For this review, take the finished solid that the model builds, in its own axes (mm). A direction names the side the tool comes from. Give positions to 0.01 mm unless a question says otherwise; leave off trailing zeros. Write each loop counter-clockwise with the first axis right and the second up, starting at its lowest first coordinate (ties: lowest second). Pieces come first, ordered by that corner, then holes.
1) We need section B-B on z = -9. Give the boundary of the cut face in (x, y).
2) Draft analysis for pull direction Z (two halves, no side actions). For faces 3 (the face through (4, 3, 0)), 4 (the face through (0, 4, 0)), 5 (the face through (1.014, -12.956, 5.122)), 6 (the face through (4.056, 10.648, -13.887)), state which applies: pulls with the +Z half, pulls with the -Z half, needs draft (parallel to the pull), parting line crosses it, or undercut.
3) Machinability: for faces 1 (the face through (1.014, 13.492, 3.472)), 2 (the face through (5.042, -15.368, -2.018)), which of the approach directions +Z, -Z, +X, -X, +Y, -Y give a long, thin tool a straight path to every point of the face, cutting with its end or side? Answer none if there is none.
4) For P1, Ø5, axis at y = -5.88, z = -8.09, coming from the -X side; P2, Ø1.5, axis at x = 6, z = -8, coming from the -Y side; P3, Ø5, axis at y = -2.5, z = 11.5, coming from the +X side; P4, Ø1, axis at x = 3.5, z = -2, coming from the +Y side, all flat-tipped, find the tip position at first contact; note any pin that passes through.
5) We need section C-C on x = 1. Give the boundary of the cut face in (y, z).
6) We need section A-A on y = 0. Give the number of separate pieces and of enclosed holes in the cut face, and give its area (3 significant figures).
7) Wall thickness on line 1 along Y through (x, z) = (3.75, 0); line 2 along Y through (x, z) = (2.25, -4.5): over which ranges is each line inside the solid? List them lowest first.
from build123d import *

# Parameters (mm, degrees)
F0_W            = 8
F0_H            = 17.5
F3_D            = 6
F4_T            = -2
F6_D            = 8
F6_COPIES_COUNT = 5
F7_SIZE         = 0.99999


# Not quite as in the source:
# - a fillet or chamfer is up to 0.001 mm smaller than in the source, because OpenCascade refuses the exact size
# - a pattern or mirror of a feature is missing from the dataset's text; its kind, count and spacing are read off the source's solid


with BuildPart() as f1:
    # F0 (on Front) → F1 (revolve)
    with BuildSketch(Plane.XZ):
        with Locations((4, 8.75)):
            Rectangle(F0_W, F0_H)
    revolve(axis=Axis((4, 0, 0), (1, 0, 0)))

    # F3 (through all)
    with Locations(Plane(origin=(0, 0, 0), x_dir=(0, 1, 0), z_dir=(-1, 0, 0))):
        with Locations((0, 0)):
            Hole(F3_D / 2)

    # F4
    f4_openings = [f1.faces().sort_by_distance(p)[0] for p in [
        (8, 0, -17.005025),
    ]]
    offset(amount=F4_T, openings=f4_openings)

    # F6 (through all)
    with Locations(Plane(origin=(0, 0, 0), x_dir=(0, 1, 0), z_dir=(-1, 0, 0))):
        with Locations((0, -10)):
            f6 = Hole(F6_D / 2)

    # F6_copies: F6 ×5 about axis
    f6_copies_axis = Axis((0, 0, 0), (1, 0, 0))
    for i in range(1, F6_COPIES_COUNT):
        add(f6.rotate(f6_copies_axis, i * 360 / F6_COPIES_COUNT), mode=Mode.SUBTRACT)

    # F7 (size 1 in the source; OpenCascade refuses exactly that, so slightly less here)
    f7_edges = [f1.edges().sort_by_distance(p)[0] for p in [
        (8, -3, 0),
        (8, -5, 0),
    ]]
    chamfer(f7_edges, length=F7_SIZE)


solid = f1.part
Results list:
1. outline: (0, -15.01) - (8, -15.01) - (8, -12.62) - (2, -12.62) - (2, -9.77) - (0, -9.77) - close; (0, -1.98) - (2, -1.98) - (2, 1.98) - (0, 1.98) - close; (0, 9.77) - (2, 9.77) - (2, 12.62) - (8, 12.62) - (8, 15.01) - (0, 15.01) - close
2. face 3: undercut
2. face 4: needs draft
2. face 5: undercut
2. face 6: parting line crosses it
3. face 1: +X, -X
3. face 2: +X
4. P1: passes through
4. P2: stops at y = -15.93
4. P3: stops at x = 2
4. P4: stops at y = 17.44
5. outline: circle Ø35 at (0, 0); hole circle Ø8 at (-9.51, 3.09); hole circle Ø8 at (-5.88, -8.09); hole circle Ø8 at (0, 10); hole circle Ø6 at (0, 0); hole circle Ø8 at (5.88, -8.09); hole circle Ø8 at (9.51, 3.09)
6. separate pieces: 3
6. enclosed holes: 0
6. area: 88.0 mm2
7. line 1: y = -17.5 to -15.5, -5 to -3, 3 to 5, 15.5 to 17.5
7. line 2: y = -16.91 to -14.83, -2.18 to 2.18, 14.83 to 16.91
